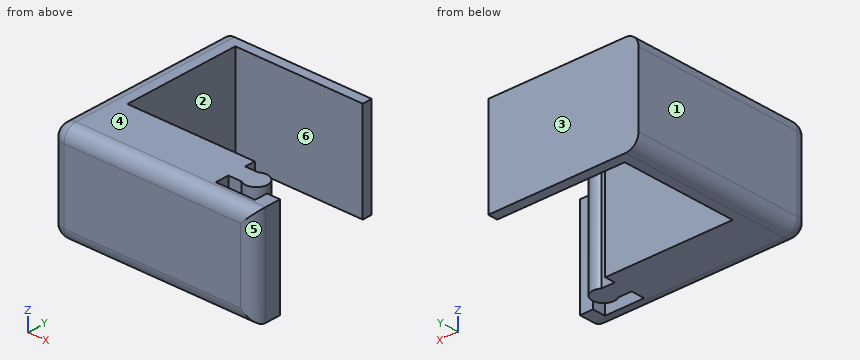
Autodesk Inventor part; units mm, degrees
ref_plane "YZ Plane" through (0, 0, 0) normal (1, 0, 0) x (0, 1, 0)
ref_plane "XZ Plane" through (0, 0, 0) normal (0, 1, 0) x (-1, 0, 0)
ref_plane "XY Plane" through (0, 0, 0) normal (0, 0, 1) x (1, 0, 0)
sketch "Эскиз1" plane through (0, 0, 0) normal (0, 0, 1) x (1, 0, 0)
  arc A0 (19.25, -13.5) -> (19.25, -10.5) centre (20.245, -12) ccw
  line L0 (19.25, -10.5) -> (17.25, -10.5)
  line L1 (17.25, -13.5) -> (19.25, -13.5)
  line L2 (17.25, -10.6) -> (19.2806, -10.6)
  arc A1 (19.2806, -13.4) -> (19.2806, -10.6) centre (20.245, -12) ccw
  line L3 (19.2806, -13.4) -> (17.25, -13.4)
  line L4 (17.25, -13.5) -> (17.25, -15.5)
  line L5 (17.25, 3) -> (17.25, -10.5)
  line L6 (19.25, -9) -> (-2.25, -9)
  line L7 (-2.25, -9) -> (-2.25, 9)
  line L8 (-2.25, 9) -> (19.25, 9)
  line L9 (17.25, 10.5) -> (17.25, 6.5)
  line L10 (17.25, 10.5) -> (-5.75, 10.5)
  line L11 (-5.75, 10.5) -> (-5.75, -17.9303)
  line L12 (23.25, -17.9303) -> (-3.75, -17.9303)
  line L13 (-5.75, -15.9303) -> (-5.75, 10.5)
  line L14 (-5.75, -17.9303) -> (-3.75, -17.9303)
  line L15 (25.25, -13.5) -> (25.25, -15.9303)
  line L16 (23.25, -13.5) -> (25.25, -13.5)
  line L17 (23.25, -15.5) -> (23.25, -13.5)
  line L18 (23.25, -17.9303) -> (-3.75, -17.9303)
  line L19 (25.25, -15.9303) -> (25.25, -17.9303)
  line L20 (25.25, -17.9303) -> (23.25, -17.9303)
  line L21 (17.25, -15.5) -> (23.25, -15.5)
  line L22 (17.25, -13.4) -> (17.25, -13.5)
  line L23 (17.25, -10.6) -> (17.25, -10.5)
  point P0 (0, 0)
  point P1 (17.25, -9)
  point P2 (17.25, 9)
  dimension "d0" = 0.1
  dimension "d1" = 23
extrude "Выдавливание1" add sketch "Эскиз1" along normal blind 15 contours L4 L21 L17 L16 L15 L19 L20 L12 L14 L11 L10 L9 L8 L7 L6 L5 L23 L2 A1 L3 L22
fillet "Сопряжение1" radius 2 6 edges at (-5.75, -17.9303, 7.5) (-5.75, -3.7151, 0) (-5.75, -3.7151, 15) (9.75, -17.9303, 0) (9.75, -17.9303, 15) (25.25, -17.9303, 7.5)
properties part number "ЛЦМК.30000.10.00.02 Крышка задняя"
Work out the finished part from the listing and answer in its coordinate system (mm). Face numbers are marked on the shaded views. A direction names the side the tool comes from. Coordinates: 2 decimals unless noted, no trailing zeros. Loops run counter-clockwise (first coordinate to the right, second up) from the corner with the lowest first, then second, coordinate; pieces in that order, holes last. Notation, with made-up numbers: (75, 81.5) -> (116, 81.5) arc R21 cw to (116, 113.5) -> close; hole circle Ø2 at (43.25, 66.5). An arc over 180 degrees is marked (long way). Write each question's results on one line, items separated by ' | '. Start each with the question number.
1) Find section D-D on x = 20. Determine the outline of the cut face in (y, z).
2) For the marked faces 1 and 2, determine the directions among +Z, -Z, +X, -X, +Y, -Y from which every point of the face is accessible in a straight line to the end or side of a thin tool.
3) Find section A-A on x = 14. Determine the outline of the cut face in (y, z), then the cut area to 3 significant figures.
4) Flat-ended cylindrical pins translate along their axes: P1, Ø1.6, axis at x = 24, z = 9.5, coming from the +Y side; P2, Ø3, axis at x = -0.5, y = -11, coming from the -Z side; P3, Ø1.5, axis at y = -5.5, z = 9.5, coming from the +X side; P4, Ø1, axis at x = 18, z = 10.5, coming from the +Y side. Find the tip coordinate at first contact, or state that the pin passes through.
5) Consider line 1 along Y through (x, z) = (-1.5, 6.5); line 2 along X through (y, z) = (-14.5, 4.75); line 3 along X through (y, z) = (-6.75, 7.25). Determine where each line is inside the solid, lowest interval first.
6) Find section C-C on y = -12. Determine the outline of the cut face in (x, z), then the cut area to 3 significant figures.
7) The mould has two halves that part along Y. Classify the marked faces 3, 4, 5 and 6: pulls with the +Y half, pulls with the -Y half, needs draft (parallel to the pull), parting line crosses it, or undercut.
Response values:
1) outline: (-17.93, 2) arc R2 ccw to (-15.93, 0) -> (-15.5, 0) -> (-15.5, 15) -> (-15.93, 15) arc R2 ccw to (-17.93, 13) -> close; (-13.68, 0) -> (-10.32, 0) -> (-10.32, 15) -> (-13.68, 15) -> close
2) face 1: +Z, -Z, -X, +Y, -Y | face 2: +Z, -Z, +X
3) outline: (-17.93, 2) arc R2 ccw to (-15.93, 0) -> (-9, 0) -> (-9, 15) -> (-15.93, 15) arc R2 ccw to (-17.93, 13) -> close; (9, 0) -> (10.5, 0) -> (10.5, 15) -> (9, 15) -> close | area: 155 mm^2
4) P1: stops at y = -13.5 | P2: stops at z = 0 | P3: stops at x = -2.25 | P4: stops at y = -10.6
5) line 1: y = -17.93 to -9, 9 to 10.5 | line 2: x = -5.75 to 17.25, 23.25 to 25.25 | line 3: x = -5.75 to -2.25
6) outline: (-5.75, 2) arc R2 ccw to (-3.75, 0) -> (21.95, 0) -> (21.95, 15) -> (-3.75, 15) arc R2 ccw to (-5.75, 13) -> close | area: 414 mm^2
7) face 3: pulls with the +Y half | face 4: needs draft | face 5: pulls with the -Y half | face 6: undercut
